Verification items for the finished model (mm, model axes). Face numbers are marked on the shaded views. A direction names the side the tool comes from. Round coordinates to 2 decimals unless told otherwise and drop trailing zeros. Order: outer loops, then holes, each group sorted by start corner. A loop starts at its lowest first (then second) coordinate and runs counter-clockwise, first axis right, second up. Notation, with made-up numbers: (-15, 45) -> (44, 45) arc R17 ccw to (44, 77) -> close; hole circle Ø7 at (54.5, -12.5). An arc over 180 degrees is marked (long way). Put each result on its own line as item: value.
```python
from build123d import *

# Parameters (mm, degrees)
BOSS_EXTRUDE1_DEPTH = 40
SKETCH2_W           = 71
SKETCH2_H           = 71
CUT_EXTRUDE1_DEPTH  = 35
SKETCH3_W           = 20
SKETCH3_H           = 8
CUT_EXTRUDE2_DEPTH  = 22.5
CIRPATTERN1_COUNT   = 2
CIRPATTERN1_ANGLE   = 90
FILLET1_R           = 4


with BuildPart() as part:
    # Sketch1 → Boss-Extrude1 (new body)
    with BuildSketch(Plane.XY):
        Polygon((0, 76), (0, 0), (76, 0), (76, 10), (10, 76), align=None)
    extrude(amount=BOSS_EXTRUDE1_DEPTH)

    # Sketch2 → Cut-Extrude1 (cut)
    with BuildSketch(Plane.XY.offset(40)):
        with Locations((40.5, 40.5)):
            Rectangle(SKETCH2_W, SKETCH2_H)
    extrude(amount=-CUT_EXTRUDE1_DEPTH, mode=Mode.SUBTRACT)

    # Sketch3 → Cut-Extrude2 (cut, symmetric)
    with BuildSketch(Plane(origin=(0, 5, 0), x_dir=(1, 0, 0), z_dir=(0, 1, 0))):
        with Locations((23, -20)):
            Rectangle(SKETCH3_W, SKETCH3_H)
        with Locations((58, -20)):
            Rectangle(SKETCH3_W, SKETCH3_H)
    cut_extrude2 = extrude(amount=CUT_EXTRUDE2_DEPTH, both=True, mode=Mode.SUBTRACT)

    # CirPattern1: Cut-Extrude2 ×2 about axis
    cirpattern1_axis = Axis((0, 0, 40), (0, 0, 1))
    for i in range(1, CIRPATTERN1_COUNT):
        add(cut_extrude2.rotate(cirpattern1_axis, i * CIRPATTERN1_ANGLE / (CIRPATTERN1_COUNT - 1)), mode=Mode.SUBTRACT)

    # Fillet1
    fillet1_edges = [part.edges().sort_by_distance(p)[0] for p in [
        (68, 2.5, 24),
        (68, 2.5, 16),
        (33, 2.5, 24),
        (33, 2.5, 16),
        (2.5, 33, 24),
        (2.5, 33, 16),
        (2.5, 68, 24),
        (2.5, 68, 16),
    ]]
    fillet(fillet1_edges, radius=FILLET1_R - 0.0001)  # a hair under: the kernel refuses the full size


solid = part.part
```
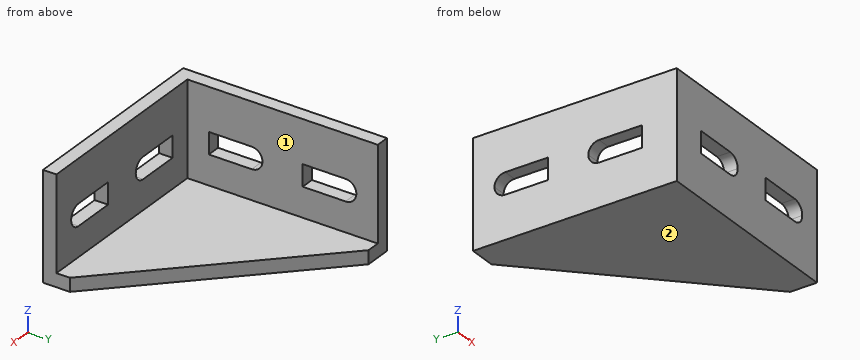
Item 1: Depth check by flat-ended pin: pin 1 Ø6 at (y, z) = (29.5, 28) entering from +X; pin 2 Ø8 at (x, z) = (43.5, 6.5) entering from +Y; pin 3 Ø2 at (y, z) = (16.5, 5) entering from +X; pin 4 Ø2.5 at (x, y) = (53.5, 3) entering from -Z. Enter the tip coordinate at first touch or a pass-through.
Geometry check:
pin 1: x = 5
pin 2: y = 46.21
pin 3: x = 70.5
pin 4: z = 0
Item 2: Tool access check on the marked faces 1 and 2. Record the directions out of +Z, -Z, +X, -X, +Y, -Y that give a thin tool (end or side, any length) a straight path to the whole face; none if there is none.
Geometry check:
face 1: +Z, +X, +Y
face 2: -Z, +X, -X, +Y, -Y
Item 3: Sectioned sample at A-A, the plane x = 20.5. Record the boundary of the cut face in (y, z).
Geometry check:
outline: (0, 0) -> (65.5, 0) -> (65.5, 5) -> (5, 5) -> (5, 16) -> (0, 16) -> close; (0, 24) -> (5, 24) -> (5, 40) -> (0, 40) -> close
Item 4: Sectioned sample at B-B, the plane y = 62.5. Record the boundary of the cut face in (x, z), then the cut area to 4 significant figures.
Geometry check:
outline: (0, 0) -> (23.5, 0) -> (23.5, 5) -> (5, 5) -> (5, 16) -> (0, 16) -> close; (0, 24) -> (5, 24) -> (5, 40) -> (0, 40) -> close
area: 252.5 mm2
Item 5: Sectioned sample at C-C, the plane z = 18. Record the boundary of the cut face in (x, y).
Geometry check:
outline: (0, 0) -> (13, 0) -> (13, 5) -> (5, 5) -> (5, 13) -> (0, 13) -> close; (0, 32.46) -> (5, 32.46) -> (5, 48) -> (0, 48) -> close; (0, 67.46) -> (5, 67.46) -> (5, 76) -> (0, 76) -> close; (32.46, 0) -> (48, 0) -> (48, 5) -> (32.46, 5) -> close; (67.46, 0) -> (76, 0) -> (76, 5) -> (67.46, 5) -> close
Item 6: Sectioned sample at D-D, the plane y = 45.5. Record the boundary of the cut face in (x, z), then the cut area to 4 significant figures.
Geometry check:
outline: (0, 0) -> (40.5, 0) -> (40.5, 5) -> (5, 5) -> (5, 40) -> (0, 40) -> close
area: 377.5 mm2
Item 7: Material ranges on line 1 along Y through (x, z) = (12.5, 35.5), recorded low to high.
Geometry check:
line 1: 0 to 5
